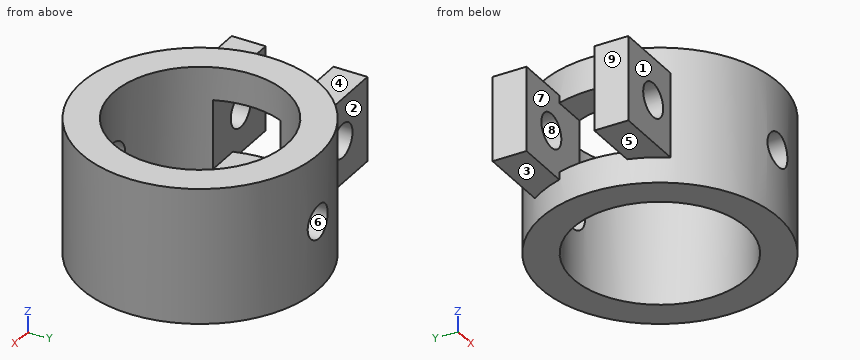
```python
from build123d import *

# Parameters (mm, degrees)
CYLINDER004_R          = 2
CYLINDER004_DEPTH      = 16
CYLINDER004_ROLL_ANGLE = -90
BOX001_W               = 5
BOX001_H               = 8
BOX001_DEPTH           = 8.2
CYLINDER006_R          = 2
CYLINDER006_DEPTH      = 30
CYLINDER006_ROLL_ANGLE = -90
CYLINDER002_R          = 10.2
CYLINDER002_DEPTH      = 28
BOX_W                  = 10
BOX_H                  = 4
BOX_DEPTH              = 10
BOX002_W               = 10
BOX002_H               = 4
BOX002_DEPTH           = 10
CYLINDER_R             = 14
CYLINDER_DEPTH         = 16


with BuildPart() as cylinder004:
    # Cylinder004 → Cylinder004 (new body)
    with BuildSketch(Plane.XY):
        Circle(CYLINDER004_R)
    extrude(amount=CYLINDER004_DEPTH)


with BuildPart() as cylinder004_1:
    # Cylinder004 roll: moved
    add(cylinder004.part.rotate(Axis((0, 0, 0), (1, 0, 0)), CYLINDER004_ROLL_ANGLE))


with BuildPart() as cylinder004_2:
    # Cylinder004 placement: moved
    add(cylinder004_1.part.moved(Location((-25, -8, 0))))


with BuildPart() as cube001:
    # Box001 → Box001 (new body)
    with BuildSketch(Plane(origin=(-24, -4, -4.1), x_dir=(1, 0, 0), z_dir=(0, 0, 1))):
        with Locations((2.5, 4)):
            Rectangle(BOX001_W, BOX001_H)
    extrude(amount=BOX001_DEPTH)


with BuildPart() as cylinder006:
    # Cylinder006 → Cylinder006 (new body)
    with BuildSketch(Plane.XY):
        Circle(CYLINDER006_R)
    extrude(amount=CYLINDER006_DEPTH)


with BuildPart() as cylinder006_1:
    # Cylinder006 roll: moved
    add(cylinder006.part.rotate(Axis((0, 0, 0), (1, 0, 0)), CYLINDER006_ROLL_ANGLE))


with BuildPart() as cylinder006_2:
    # Cylinder006 placement: moved
    add(cylinder006_1.part.moved(Location((-10, -15, 0))))


with BuildPart() as negative_fusion:
    # Cylinder002 → Cylinder002 (new body)
    with BuildSketch(Plane(origin=(-10, 0, -10), x_dir=(1, 0, 0), z_dir=(0, 0, 1))):
        Circle(CYLINDER002_R)
    extrude(amount=CYLINDER002_DEPTH)

    # Fusion001: union Cylinder004, Cube001, Cylinder006
    add(cylinder004_2.part)
    add(cube001.part)
    add(cylinder006_2.part)


with BuildPart() as cube:
    # Box → Box (new body)
    with BuildSketch(Plane(origin=(-30, -8, -5), x_dir=(1, 0, 0), z_dir=(0, 0, 1))):
        with Locations((5, 2)):
            Rectangle(BOX_W, BOX_H)
    extrude(amount=BOX_DEPTH)


with BuildPart() as cube002:
    # Box002 → Box002 (new body)
    with BuildSketch(Plane(origin=(-30, 4, -5), x_dir=(1, 0, 0), z_dir=(0, 0, 1))):
        with Locations((5, 2)):
            Rectangle(BOX002_W, BOX002_H)
    extrude(amount=BOX002_DEPTH)


with BuildPart() as cut:
    # Cylinder → Cylinder (new body)
    with BuildSketch(Plane(origin=(-10, 0, -8), x_dir=(1, 0, 0), z_dir=(0, 0, 1))):
        Circle(CYLINDER_R)
    extrude(amount=CYLINDER_DEPTH)

    # Fusion: union Cube, Cube002
    add(cube.part)
    add(cube002.part)

    # Cut: cut Negative Fusion
    add(negative_fusion.part, mode=Mode.SUBTRACT)


solid = cut.part
```
Verification items for the finished model (mm, model axes). Face numbers are marked on the shaded views. A direction names the side the tool comes from. Coordinates: 2 decimals unless noted, no trailing zeros. Loops run counter-clockwise (first coordinate to the right, second up) from the corner with the lowest first, then second, coordinate; pieces in that order, holes last. Notation, with made-up numbers: (42, -35) - (87, -35) arc R13 cw to (87, -27) - close; hole circle Ø11 at (32.25, -18). An arc over 180 degrees is marked (long way). Put each result on its own line as item: value.
Item 1: Scan lines: line 1 along X through (y, z) = (-5.25, -1.5); line 2 along Z through (x, y) = (-20.5, -3.75); line 3 along Z through (x, y) = (-10, -12.7). Record each from-to range of solid material in increasing order.
Conclusion:
line 1: x = -30 to -26.32, -23.68 to -18.75, -1.25 to 2.98
line 2: z = -8 to -4.1, 4.1 to 8
line 3: z = -8 to -2, 2 to 8
Item 2: Section check D-D (x = -17). Enter the section's corners in (y, z).
Conclusion:
outline: (-12.12, -8) - (-7.42, -8) - (-7.42, 8) - (-12.12, 8) - close; (7.42, -8) - (12.12, -8) - (12.12, 8) - (7.42, 8) - close
Item 3: Gauge pin test, flat ends, axial feed: pin 1 Ø4.5 at (x, z) = (-27.5, 2) entering from +Y; pin 2 Ø2 at (y, z) = (-10, -4.5) entering from +X; pin 3 Ø8 at (x, z) = (-2.5, -5) entering from +Y. Record the tip position at first contact, or that the pin passes through.
Conclusion:
pin 1: stops at y = 8
pin 2: stops at x = 0.72
pin 3: stops at y = 13.56
Item 4: Set-up check for the marked faces 1, 2, 3, 4 and 5: record each of +Z, -Z, +X, -X, +Y, -Y from which the full face is reachable in a straight line by a thin tool's end or side.
Conclusion:
face 1: +Z, -Z, -X, -Y
face 2: +Z, -Z, -X, +Y
face 3: -Z, -X, +Y
face 4: +Z, -X, +Y
face 5: -Z, -X, -Y
Item 5: Section check C-C (y = -4.5). Enter the section's corners in (x, z), then the cut area to 3 significant figures.
Conclusion:
outline: (-30, -5) - (-23.26, -5) - (-23.26, -8) - (-19.15, -8) - (-19.15, 8) - (-23.26, 8) - (-23.26, 5) - (-30, 5) - close; (-0.85, -8) - (3.26, -8) - (3.26, 8) - (-0.85, 8) - close; hole circle Ø4 at (-25, 0)
area: 186 mm2
Item 6: Draft check along X on the marked faces 6, 7, 8 and 9. Enter one of: pulls with the +X half, pulls with the -X half, needs draft (parallel to the pull), parting line crosses it, or undercut.
Conclusion:
face 6: undercut
face 7: needs draft
face 8: undercut
face 9: pulls with the -X half
Item 7: Section check A-A (y = 0). Enter the section's corners in (x, z).
Conclusion:
outline: (-24, -8) - (-20.2, -8) - (-20.2, -4.1) - (-24, -4.1) - close; (-24, 4.1) - (-20.2, 4.1) - (-20.2, 8) - (-24, 8) - close; (0.2, -8) - (4, -8) - (4, 8) - (0.2, 8) - close
Item 8: Section check B-B (x = -10). Enter the section's corners in (y, z).
Conclusion:
outline: (-14, -8) - (-10.2, -8) - (-10.2, -2) - (-14, -2) - close; (-14, 2) - (-10.2, 2) - (-10.2, 8) - (-14, 8) - close; (10.2, -8) - (14, -8) - (14, -2) - (10.2, -2) - close; (10.2, 2) - (14, 2) - (14, 8) - (10.2, 8) - close
